Read the model definition and answer for the solid it produces. Units are mm, in the model's axes. Coordinates: 2 decimals unless noted, no trailing zeros. Write each loop counter-clockwise with the first axis right and the second up, starting at its lowest first coordinate (ties: lowest second). Pieces come first, ordered by that corner, then holes.
(1) Given pin 1 (3 mm diameter, centred on y = 10, z = 7, fed in from +X); pin 2 (12 mm diameter, centred on x = 17.5, y = -10, fed in from -Z); pin 3 (5 mm diameter, centred on x = 19.5, z = 3, fed in from +Y), each flat-ended and moving along its own axis, determine where each tip first touches the part or whether it passes through.
(2) Find the intervals of material crossed by probe 1 along X at (y, z) = (5, 6); probe 2 along X at (y, z) = (11, 6.5); probe 3 along Y at (x, z) = (-7, 1.75), in increasing order.
(3) Section A-A on z = 4 is taken. Write down the section's boundary in (x, y), then the cut area to 3 significant figures.
(4) Section B-B on x = -20 is taken. Write down the section's boundary in (y, z).
(5) Section C-C on y = 22 is taken. Write down the section's boundary in (x, z), then the cut area to 3 significant figures.
from build123d import *

# Parameters (mm, degrees)
F0_W     = 50
F0_H     = 100
F1_DEPTH = 10
F2_SIZE  = 10
F4_DEPTH = 10.001


with BuildPart() as f1:
    # F0 (on Top) → F1 (new body)
    with BuildSketch(Plane.XY):
        Rectangle(F0_W, F0_H)
    extrude(amount=F1_DEPTH)

    # F2
    f2_edges = [f1.edges().sort_by_distance(p)[0] for p in [
        (-25, -50, 5),
    ]]
    chamfer(f2_edges, length=F2_SIZE)

    # F3 (on face) → F4 (cut, through all)
    with BuildSketch(Plane.XY.offset(10)):
        Polygon((25, 50), (-15, 50), (25, -40), align=None)
    extrude(amount=-F4_DEPTH, mode=Mode.SUBTRACT)


solid = f1.part
Response:
1. pin 1: stops at x = 3.44
1. pin 2: stops at z = 0
1. pin 3: stops at y = -22
2. probe 1: x = -25 to 5
2. probe 2: x = -25 to 2.33
2. probe 3: y = -50 to 32
3. outline: (-25, -40) - (-15, -50) - (25, -50) - (25, -40) - (-15, 50) - (-25, 50) - close
3. area: 3,150 mm2
4. outline: (-45, 0) - (50, 0) - (50, 10) - (-45, 10) - close
5. outline: (-25, 0) - (-2.56, 0) - (-2.56, 10) - (-25, 10) - close
5. area: 224 mm2
